Read the model definition and answer for the solid it produces. Units are mm, in the model's axes. A direction names the side the tool comes from. Coordinates: 2 decimals unless noted, no trailing zeros. Write each loop counter-clockwise with the first axis right and the second up, starting at its lowest first coordinate (ties: lowest second). Pieces come first, ordered by that corner, then holes.
1) Find the intervals of material crossed by line 1 (Z direction, x = 22, y = 4.25); line 2 (Y direction, x = 1.5, z = 10.5), in increasing order.
2) The part is cut by section A-A (y = 6). Determine the outline of the cut face in (x, z).
3) Which of the six approach directions +Z, -Z, +X, -X, +Y, -Y give full straight-line access (tool end or side, diameter ignored) to faces 1 (the face through (18, 5, -0.7)), 2 (the face through (11, 0, 11)), 3 (the face through (-0.7, 5, 17))?
4) The part is cut by section D-D (x = 1.5). Determine the outline of the cut face in (y, z), then the cut area to 3 significant figures.
5) The part is cut by section B-B (x = 28). Determine the outline of the cut face in (y, z), then the cut area to 3 significant figures.
6) Each of these flat-tipped pins is pushed along its axis until it touches: pin 1 Ø9 at (x, z) = (10.5, 10) entering from +Y; pin 2 Ø1.1 at (x, y) = (-0.5, 2) entering from -Z; pin 3 Ø1.1 at (y, z) = (3, -1) entering from -X. Where does it stop, or does it pass through?
7) The part is cut by section C-C (z = 12.5). Determine the outline of the cut face in (x, y), then the cut area to 3 significant figures.
from build123d import *

# Parameters (mm, degrees)
BASE_FLANGE1_DEPTH      = 0.7
BREAK_CORNER1_OUTLINE_W = 10
BREAK_CORNER1_OUTLINE_H = 3
BREAK_CORNER1_DEPTH     = 3.535533906
EDGE_FLANGE2_DEPTH      = 25
EDGE_FLANGE2_BEND_DEPTH = 25


# Read off the part's stored shape, not the designer's step: Break-Corner1
# Sheet-metal steps are written as plain solids
with BuildPart() as part:
    # Sketch2 → Base-Flange1 (new body)
    with BuildSketch(Plane(origin=(0, 0, 0), x_dir=(1, 0, 0), z_dir=(0, 1, 0))):
        Polygon((0, 0), (0, -30), (30, 0), align=None)
    extrude(amount=-BASE_FLANGE1_DEPTH)

    # Break-Corner1 outline → Break-Corner1 (cut)
    with BuildSketch(Plane(origin=(0, 0, 0), x_dir=(0.7071067811865471, 0, -0.707106781186548), z_dir=(0.707106781186548, 0, 0.707106781186547))):
        with Locations((0, -0.5)):
            Rectangle(BREAK_CORNER1_OUTLINE_W, BREAK_CORNER1_OUTLINE_H)
    extrude(amount=BREAK_CORNER1_DEPTH, mode=Mode.SUBTRACT)

    # Edge-Flange2 section (across the edge) → Edge-Flange2 (add)
    with BuildSketch(Plane(origin=(-0.7, 0, 5), x_dir=(1, 0, 0), z_dir=(0, 0, 1))):
        with BuildLine():
            Line((-0.7, 0.7), (-0.7, 10))
            Line((-0.7, 10), (0, 10))
            Line((0, 10), (0, 0.7))
            ThreePointArc((0, 0.7), (0.205025253, 0.205025253), (0.7, 0))
            Line((0.7, 0), (0.7, -0.7))
            ThreePointArc((0.7, -0.7), (-0.289949494, -0.289949494), (-0.7, 0.7))
        make_face()
    extrude(amount=EDGE_FLANGE2_DEPTH)

    # Edge-Flange2 section 2 (across the edge) → Edge-Flange2 bend (add)
    with BuildSketch(Plane(origin=(30, 0, -0.7), x_dir=(0, 0, 1), z_dir=(-1, 0, 0))):
        with BuildLine():
            Line((-0.7, 0.7), (-0.7, 10))
            Line((-0.7, 10), (0, 10))
            Line((0, 10), (0, 0.7))
            ThreePointArc((0, 0.7), (0.205025253, 0.205025253), (0.7, 0))
            Line((0.7, 0), (0.7, -0.7))
            ThreePointArc((0.7, -0.7), (-0.289949494, -0.289949494), (-0.7, 0.7))
        make_face()
    extrude(amount=EDGE_FLANGE2_BEND_DEPTH)


solid = part.part
Reported:
1. line 1: z = -1.4 to -0.7
1. line 2: y = -0.7 to 0
2. outline: (-1.4, 5) - (-0.7, 5) - (-0.7, 30) - (-1.4, 30) - close; (5, -1.4) - (30, -1.4) - (30, -0.7) - (5, -0.7) - close
3. face 1: +Z, +X, -X, +Y
3. face 2: +Z, +X, +Y
3. face 3: +Z, -Z, +X, +Y
4. outline: (-0.7, 3.5) - (0, 3.5) - (0, 28.5) - (-0.7, 28.5) - close
4. area: 17.5 mm2
5. outline: (-0.7, 0) arc R1.4 ccw to (0.7, -1.4) - (10, -1.4) - (10, -0.7) - (0.7, -0.7) arc R0.7 cw to (0, 0) - (0, 2) - (-0.7, 2) - close
5. area: 9.06 mm2
6. pin 1: stops at y = 0
6. pin 2: stops at z = 5
6. pin 3: stops at x = 5
7. outline: (-1.4, 0.7) arc R1.4 ccw to (0, -0.7) - (17.5, -0.7) - (17.5, 0) - (0, 0) arc R0.7 cw to (-0.7, 0.7) - (-0.7, 10) - (-1.4, 10) - close
7. area: 19.9 mm2
